Source: CAD feature listing. Evaluate the final solid. Frame: model axes, mm. A direction names the side the tool comes from. Coordinates: 2 decimals unless noted, no trailing zeros. Order: outer loops, then holes, each group sorted by start corner. A loop starts at its lowest first (then second) coordinate and runs counter-clockwise, first axis right, second up. Notation, with made-up numbers: (54, 66) - (110, 66) arc R25 ccw to (110, 86) - close; hole circle Ø2 at (34.5, -19). An arc over 180 degrees is marked (long way). One line per question, with ' | ' between items.
from build123d import *

# Parameters (mm, degrees)
SKIZZE1_R                       = 1.75
AUFSATZ_LINEAR_AUSTRAGEN1_DEPTH = 10
SKIZZE2_W                       = 14
SKIZZE2_H                       = 25
AUFSATZ_LINEAR_AUSTRAGEN2_DEPTH = 2
VERRUNDUNG5_R                   = 3
VERRUNDUNG6_R                   = 5
VERRUNDUNG7_R                   = 1


with BuildPart() as part:
    # Skizze1 → Aufsatz-Linear austragen1 (new body)
    with BuildSketch(Plane.XY):
        Polygon((0, 0), (0, 47), (-5.100622615, 47), (-22.207223625, 0), align=None)
        with Locations((-3, 44)):
            Circle(SKIZZE1_R, mode=Mode.SUBTRACT)
    extrude(amount=AUFSATZ_LINEAR_AUSTRAGEN1_DEPTH)

    # Skizze2 → Aufsatz-Linear austragen2 (add)
    with BuildSketch(Plane(origin=(0, 0, 0), x_dir=(0, 0, -1), z_dir=(1, 0, 0))):
        with Locations((-5, 12.5)):
            Rectangle(SKIZZE2_W, SKIZZE2_H)
    extrude(amount=AUFSATZ_LINEAR_AUSTRAGEN2_DEPTH)

    # Verrundung5
    verrundung5_edges = [part.edges().sort_by_distance(p)[0] for p in [
        (-5.100622615, 47, 5),
        (0, 47, 5),
    ]]
    fillet(verrundung5_edges, radius=VERRUNDUNG5_R - 0.0001)  # a hair under: the kernel refuses the full size

    # Verrundung6
    verrundung6_edges = [part.edges().sort_by_distance(p)[0] for p in [
        (-22.207223625, 0, 5),
    ]]
    fillet(verrundung6_edges, radius=VERRUNDUNG6_R)

    # Verrundung7
    verrundung7_edges = [part.edges().sort_by_distance(p)[0] for p in [
        (-4.720741972, 46.457474218, 0),
        (-0.878650367, 46.121349633, 0),
        (0, 34.50005, 0),
        (0, 34.50005, 10),
        (-4.720741972, 46.457474218, 10),
        (-0.878650367, 46.121349633, 10),
        (-19.162243813, 2.132117818, 0),
        (-19.162243813, 2.132117818, 10),
        (-7.533241796, 0, 10),
        (-7.533241796, 0, 0),
        (-12.792000305, 25.868113472, 0),
        (-12.792000305, 25.868113472, 10),
    ]]
    fillet(verrundung7_edges, radius=VERRUNDUNG7_R)


solid = part.part
(1) Pin query (flat end, axial travel): P1, Ø5.5, axis at x = -11.5, y = 28.5, coming from the +Z side; P2, Ø2, axis at y = 10.5, z = 2, coming from the -X side; P3, Ø1, axis at y = 38, z = 0.5, coming from the -X side. Return the tip coordinate at first contact, or that it passes through.
Taken from the geometry:
P1: stops at z = 10 | P2: stops at x = -18.75 | P3: stops at x = -8.5
(2) Cut plane B-B (z = 11). Return the cut outline in (x, y), and give its area (3 significant figures).
Taken from the geometry:
outline: (0, 0) - (2, 0) - (2, 25) - (0, 25) - close | area: 50.0 mm²
(3) Material intervals for L1, parallel to Y at x = -3, z = 3.5; L2, parallel to Z at x = -3, y = 22; L3, parallel to Y at x = 1, z = 8.25, sorted ascending. Write a range as from..to.
Taken from the geometry:
L1: y = 0..42.25, 45.75..47 | L2: z = 0..10 | L3: y = 0..25
(4) Set-up query: faces 1 (the flat face through (-8, 19, 10)), 2 (the flat face through (0, 34, 5)), 3 (the cylindrical face through (-12.62, 25.5, 9.7)), 4 (the cylindrical face through (-0.285, 34.633, 9.699)), 5 (the cylindrical face through (-7.428, 0.285, 9.699)). Return all of +Z, -Z, +X, -X, +Y, -Y with unobstructed straight access to the full face (end or side cutting, diameter ignored); none if empty.
Taken from the geometry:
face 1: +Z, -X, +Y, -Y | face 2: +Z, -Z, +X, +Y | face 3: +Z, -X, +Y | face 4: +Z, +X, +Y | face 5: +Z, -X, -Y
(5) Pull-direction query (Y, two-part tool) for faces 6 (the flat face through (1, 25, 5)), 7 (the flat face through (-8, 19, 0)), 8 (the cylindrical face through (-7.639, 0.301, 0.285)), 9 (the cylindrical face through (-3.38, 42.29, 4.93)); classes: pulls with the +Y half, pulls with the -Y half, needs draft (parallel to the pull), parting line crosses it, or undercut.
Taken from the geometry:
face 6: pulls with the +Y half | face 7: needs draft | face 8: pulls with the -Y half | face 9: undercut
